Verification items for the finished model (mm, model axes). Face numbers are marked on the shaded views. A direction names the side the tool comes from. Round coordinates to 2 decimals unless told otherwise and drop trailing zeros. Write each loop counter-clockwise with the first axis right and the second up, starting at its lowest first coordinate (ties: lowest second). Pieces come first, ordered by that corner, then holes.
from build123d import *

# Parameters (mm, degrees)
BOSS_EXTRUDE1_DEPTH      = 2.5
BOSS_EXTRUDE2_DEPTH      = 1.5
BOSS_EXTRUDE2_DEPTH_BACK = 1.5
FILLET1_R                = 1.5
SKETCH5_W                = 5
SKETCH5_H                = 10
BOSS_EXTRUDE3_DEPTH      = 7.5
SKETCH6_R                = 3
CUT_EXTRUDE1_DEPTH       = 2.5
CUT_EXTRUDE2_DEPTH       = 2.5
FILLET2_R                = 3
CUT_EXTRUDE3_DEPTH       = 10


with BuildPart() as part:
    # Sketch1 → Boss-Extrude1 (new body)
    with BuildSketch(Plane(origin=(0, 0, 0), x_dir=(1, 0, 0), z_dir=(0, 1, 0))):
        with BuildLine():
            Line((-20.209371097, 50.622586501), (-32.257467167, 50.622586501))
            ThreePointArc((-32.257467167, 50.622586501), (-33.362688598, 43.122586501), (-32.257467167, 35.622586501))
            Line((-32.257467167, 35.622586501), (-20.209371097, 35.622586501))
            Line((-20.209371097, 35.622586501), (-12.362688598, 37.872586501))
            Line((-12.362688598, 37.872586501), (-12.362688598, 48.372586501))
            Line((-12.362688598, 48.372586501), (-20.209371097, 50.622586501))
        make_face()
        with BuildLine():
            Line((-32.257467167, 50.622586501), (-34.339530518, 50.622586501))
            ThreePointArc((-34.339530518, 50.622586501), (-35.362688598, 43.122586501), (-34.339530518, 35.622586501))
            Line((-34.339530518, 35.622586501), (-32.257467167, 35.622586501))
            ThreePointArc((-32.257467167, 35.622586501), (-33.362688598, 43.122586501), (-32.257467167, 50.622586501))
        make_face()
    extrude(amount=BOSS_EXTRUDE1_DEPTH)

    # Sketch4 → Boss-Extrude2 (add, two sides)
    with BuildSketch(Plane.XZ) as boss_extrude2_sk:
        with BuildLine():
            Line((-19.362688598, -38.122586501), (-32.877390242, -38.122586501))
            ThreePointArc((-32.877390242, -38.122586501), (-33.362688598, -43.122586501), (-32.877390242, -48.122586501))
            Line((-32.877390242, -48.122586501), (-19.362688598, -48.122586501))
            Line((-19.362688598, -48.122586501), (-19.362688598, -38.122586501))
        make_face()
    extrude(amount=BOSS_EXTRUDE2_DEPTH)
    extrude(boss_extrude2_sk.sketch, amount=-BOSS_EXTRUDE2_DEPTH_BACK)

    # Fillet1
    fillet1_edges = [part.edges().sort_by_distance(p)[0] for p in [
        (-27.274450808, 2.5, -35.622586501),
        (-16.286029847, 2.5, -36.747586501),
        (-12.362688598, 2.5, -43.122586501),
        (-16.286029847, 2.5, -49.497586501),
        (-27.274450808, 2.5, -50.622586501),
        (-35.362688598, 2.5, -43.122586501),
    ]]
    fillet(fillet1_edges, radius=FILLET1_R)

    # Sketch5 → Boss-Extrude3 (add)
    with BuildSketch(Plane.XZ.offset(1.5)):
        with Locations((-21.862688598, -43.122586501)):
            Rectangle(SKETCH5_W, SKETCH5_H)
    extrude(amount=BOSS_EXTRUDE3_DEPTH)

    # Sketch6 → Cut-Extrude1 (cut)
    with BuildSketch(Plane(origin=(-19.362688598, 0, 0), x_dir=(0, 0, -1), z_dir=(1, 0, 0))):
        with Locations((43.122586501, -5)):
            Circle(SKETCH6_R)
    extrude(amount=-CUT_EXTRUDE1_DEPTH, mode=Mode.SUBTRACT)

    # Sketch7 → Cut-Extrude2 (cut)
    with BuildSketch(Plane(origin=(-21.862688598, 0, 0), x_dir=(0, 0, -1), z_dir=(1, 0, 0))):
        with BuildLine():
            Line((45.84976453, -3.75), (40.395408473, -3.75))
            ThreePointArc((40.395408473, -3.75), (40.122586501, -5), (40.395408473, -6.25))
            Line((40.395408473, -6.25), (45.84976453, -6.25))
            ThreePointArc((45.84976453, -6.25), (46.053587532, -5.639713183), (46.122586501, -5))
            ThreePointArc((46.122586501, -5), (46.053587532, -4.360286817), (45.84976453, -3.75))
        make_face()
    extrude(amount=-CUT_EXTRUDE2_DEPTH, mode=Mode.SUBTRACT)

    # Fillet2
    fillet2_edges = [part.edges().sort_by_distance(p)[0] for p in [
        (-21.862688598, -9, -38.122586501),
        (-21.862688598, -9, -48.122586501),
    ]]
    fillet(fillet2_edges, radius=FILLET2_R)

    # Sketch8 → Cut-Extrude3 (cut)
    with BuildSketch(Plane.XZ):
        with BuildLine():
            Line((-19.362688598, -48.122586501), (-19.362688598, -38.122586501))
            Line((-19.362688598, -38.122586501), (-32.877390242, -38.122586501))
            ThreePointArc((-32.877390242, -38.122586501), (-33.362688598, -43.122586501), (-32.877390242, -48.122586501))
            Line((-32.877390242, -48.122586501), (-19.362688598, -48.122586501))
        make_face()
        with BuildLine():
            Line((-19.612688598, -47.872586501), (-19.612688598, -38.372586501))
            Line((-19.612688598, -38.372586501), (-32.670790068, -38.372586501))
            ThreePointArc((-32.670790068, -38.372586501), (-33.112688598, -43.122586501), (-32.670790068, -47.872586501))
            Line((-32.670790068, -47.872586501), (-19.612688598, -47.872586501))
        make_face(mode=Mode.SUBTRACT)
    extrude(amount=CUT_EXTRUDE3_DEPTH, mode=Mode.SUBTRACT)


solid = part.part
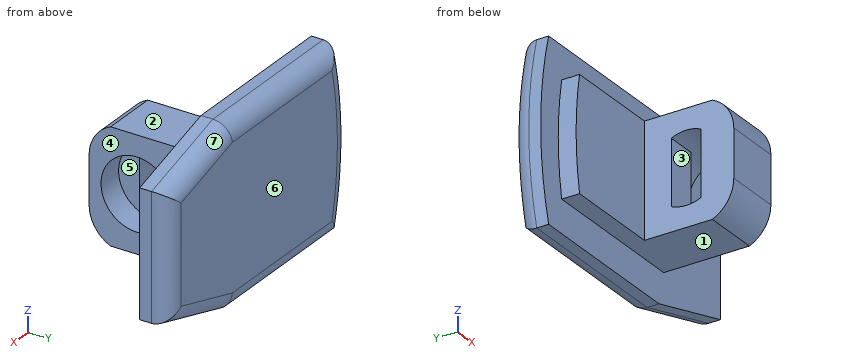
Q1. Sectioned sample at D-D (y = -2.75). Enter the section's corners in (x, z).
Recorded:
outline: (-24.36, -47.87) - (-19.61, -47.87) - (-19.61, -45.11) - (-21.86, -45.11) - (-21.86, -41.14) - (-19.61, -41.14) - (-19.61, -38.37) - (-24.36, -38.37) - close
Q2. Sectioned sample at A-A (y = -4). Enter the section's corners in (x, z).
Recorded:
outline: (-24.36, -47.87) - (-19.61, -47.87) - (-19.61, -45.95) - (-24.36, -45.95) - close; (-24.36, -40.29) - (-19.61, -40.29) - (-19.61, -38.37) - (-24.36, -38.37) - close
Q3. Material ranges on line 1 along Z through (x, y) = (-20.85, -5); line 2 along Y through (x, z) = (-15, -43.5); line 3 along Z through (x, y) = (-22.25, -0.25), recorded low to high.
Recorded:
line 1: z = -47.87 to -46.12, -40.12 to -38.37
line 2: y = 0 to 2.5
line 3: z = -47.87 to -38.37
Q4. Depth check by flat-ended pin: P1, Ø5, axis at x = -28, z = -42.5, coming from the -Y side; P2, Ø2, axis at y = -4, z = -44, coming from the -X side; P3, Ø1, axis at x = -23.5, y = -7.5, coming from the -Z side. Enter the tip coordinate at first touch or a pass-through.
Recorded:
P1: stops at y = -1.5
P2: stops at x = -24.36
P3: stops at z = -47.87
Q5. Tool access check on the marked faces 1, 2, 3 and 4. Record the directions out of +Z, -Z, +X, -X, +Y, -Y that give a thin tool (end or side, any length) a straight path to the whole face; none if there is none.
Recorded:
face 1: -Z, +X, -X, -Y
face 2: +Z, +X, -X, -Y
face 3: +X, -X
face 4: +Z, -Z, +X, -Y
Q6. Sectioned sample at B-B (x = -26.25). Enter the section's corners in (y, z), plus the area to 3 significant figures.
Recorded:
outline: (-1.5, -47.87) - (0, -47.87) - (0, -50.62) - (1, -50.62) arc R1.5 ccw to (2.5, -49.12) - (2.5, -37.12) arc R1.5 ccw to (1, -35.62) - (0, -35.62) - (0, -38.37) - (-1.5, -38.37) - close
area: 50.8 mm2
Q7. Sectioned sample at C-C (y = 0.25). Enter the section's corners in (x, z), plus the area to 3 significant figures.
Recorded:
outline: (-34.34, -50.62) - (-20.21, -50.62) - (-12.36, -48.37) - (-12.36, -37.87) - (-20.21, -35.62) - (-34.34, -35.62) arc R28 ccw to start
area: 322 mm2
Q8. Release check for a two-part mould opening along Z. For the marked faces 5, 6 and 7 record: released by +Z, released by -Z, zero draft, split by the parting line, or undercut.
Recorded:
face 5: undercut
face 6: zero draft
face 7: released by +Z
